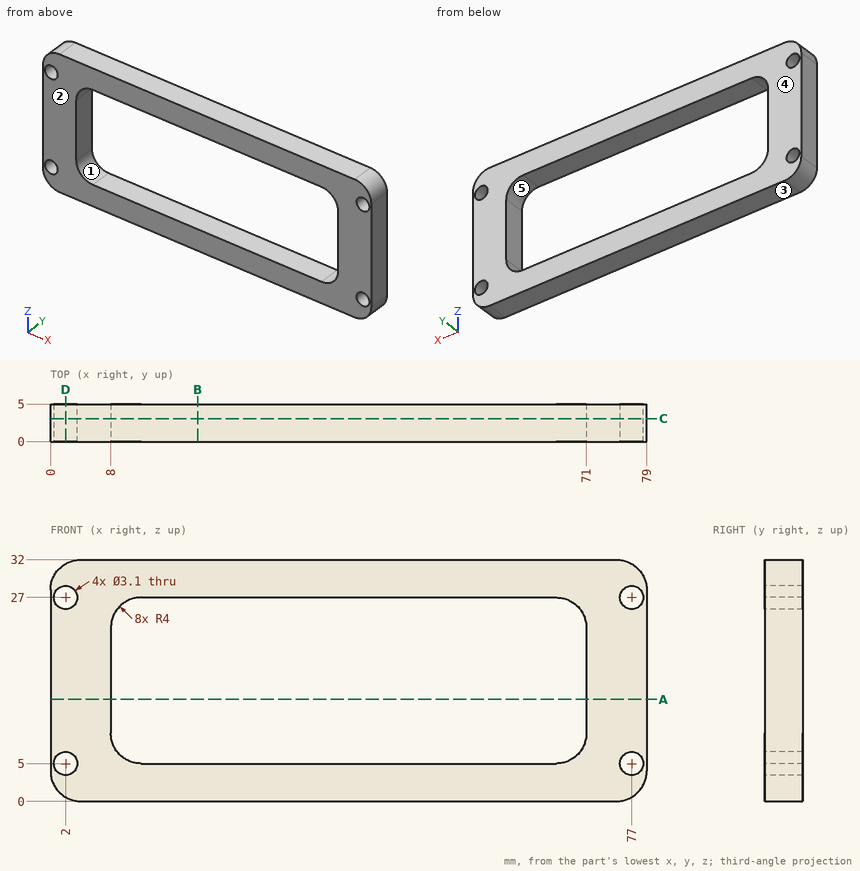
Study the drawing (mm; zero at the part's minimum x, y, z) and answer. A direction names the side the tool comes from. Round coordinates to 2 decimals unless told otherwise and drop trailing zeros. Write each loop counter-clockwise with the first axis right and the second up, starting at its lowest first coordinate (ties: lowest second). Pieces come first, ordered by that corner, then holes. Notation, with made-up numbers: (68, -26) -> (104, -26) arc R14 ccw to (104, -9) -> close; hole circle Ø6 at (68.25, 27.25). An arc over 180 degrees is marked (long way). Answer as CSV lines item,"result". Start each with the question number.
(1) The part is cut by section A-A, the plane z = 13.5. Give the vertices of the cut face in (x, y), then the cut area to 3 significant figures.
(2) A tool of negligible diameter and unlimited length cuts with its end or side. For the marked faces 4 and 5, from which of +Z, -Z, +X, -X, +Y, -Y can it reach the whole face along a straight path? Write none if from no direction.
(3) Each of these flat-tipped pins is pushed along its axis until it touches: pin 1 (3 mm diameter, centred on x = 2, z = 27, fed in from -Y); pin 2 (4 mm diameter, centred on x = 2, z = 5, fed in from -Y). Where does it stop, or does it pass through?
(4) Find the intervals of material crossed by probe 1 along Z at (x, y) = (77, 3.8); probe 2 along Z at (x, y) = (58, 1.95); probe 3 along X at (y, z) = (0.95, 19.5), in increasing order.
(5) The part is cut by section C-C, the plane y = 3.05. Give the vertices of the cut face in (x, z), then the cut area to 3 significant figures.
(6) The part is cut by section D-D, the plane x = 2. Give the vertices of the cut face in (y, z), then the cut area to 3 significant figures.
(7) The mould has two halves that part along Z. Classify the marked faces 1, 2 and 3: +Z half, -Z half, draft (parallel to the pull), parting line (faces both ways), or undercut.
(8) The part is cut by section B-B, the plane x = 19.5. Give the vertices of the cut face in (y, z).
Output values:
1,outline,"(0, 0) -> (8, 0) -> (8, 5) -> (0, 5) -> close; (71, 0) -> (79, 0) -> (79, 5) -> (71, 5) -> close"
1,area,"80.0 mm²"
2,face 4,"+Z, -Z, +X, -X, +Y"
2,face 5,"+Y, -Y"
3,pin 1,"passes through"
3,pin 2,"stops at y = 0"
4,probe 1,"z = 0.54 to 3.45, 6.55 to 25.45, 28.55 to 31.46"
4,probe 2,"z = 0 to 5, 27 to 32"
4,probe 3,"x = 0 to 8, 71 to 79"
5,outline,"(0, 4) arc R4 ccw to (4, 0) -> (75, 0) arc R4 ccw to (79, 4) -> (79, 28) arc R4 ccw to (75, 32) -> (4, 32) arc R4 ccw to (0, 28) -> close; hole circle Ø3.1 at (2, 5); hole circle Ø3.1 at (2, 27); hole (8, 9) arc R4 ccw to (12, 5) -> (67, 5) arc R4 ccw to (71, 9) -> (71, 23) arc R4 ccw to (67, 27) -> (12, 27) arc R4 ccw to (8, 23) -> close; hole circle Ø3.1 at (77, 5); hole circle Ø3.1 at (77, 27)"
5,area,"1,110 mm²"
6,outline,"(0, 0.54) -> (5, 0.54) -> (5, 3.45) -> (0, 3.45) -> close; (0, 6.55) -> (5, 6.55) -> (5, 25.45) -> (0, 25.45) -> close; (0, 28.55) -> (5, 28.55) -> (5, 31.46) -> (0, 31.46) -> close"
6,area,"124 mm²"
7,face 1,"undercut"
7,face 2,"draft"
7,face 3,"-Z half"
8,outline,"(0, 0) -> (5, 0) -> (5, 5) -> (0, 5) -> close; (0, 27) -> (5, 27) -> (5, 32) -> (0, 32) -> close"
